from build123d import *

# Parameters (mm, degrees)
FILLET1_R = 0.5


with BuildPart() as part:
    # Sketch1 → Revolve1 (revolve)
    with BuildSketch(Plane.XY):
        with BuildLine():
            Line((10, 0), (10, 26.585564127))
            Line((10, 26.585564127), (1.265397394, 28.234602606))
            Line((1.265397394, 28.234602606), (0, 29.5))
            Line((0, 29.5), (0, 30))
            Line((0, 30), (0.2, 30))
            ThreePointArc((0.2, 30), (0.225652916, 29.998347997), (0.250882045, 29.993419279))
            Line((0.250882045, 29.993419279), (0.8, 29.848964991))
            Line((0.8, 29.848964991), (10.685516518, 27.982641146))
            ThreePointArc((10.685516518, 27.982641146), (11.269907955, 27.638154951), (11.5, 27))
            Line((11.5, 27), (11.5, 0))
            Line((11.5, 0), (10, 0))
        make_face()
    revolve(axis=Axis((0, 9.5, 0), (0, -1, 0)))

    # Fillet1
    fillet1_edges = [part.edges().sort_by_distance(p)[0] for p in [
        (-0.8, 29.848964991, 0),
        (-11.5, 0, 0),
        (-10, 0, 0),
    ]]
    fillet(fillet1_edges, radius=FILLET1_R)


solid = part.part
Geometry: final body of the model. Coordinates: model frame, mm. A direction names the side the tool comes from. Give positions to 0.01 mm unless a question says otherwise; leave off trailing zeros. Write each loop counter-clockwise with the first axis right and the second up, starting at its lowest first coordinate (ties: lowest second). Pieces come first, ordered by that corner, then holes. Notation, with made-up numbers: (10.5, -6) -> (24.5, -6) arc R19 ccw to (24.5, 26) -> close; hole circle Ø3 at (-18.75, 1.25). An arc over 180 degrees is marked (long way). Answer as a JSON object with one key per item and string values.
1. Cut plane A-A on y = 4.5. Output: boundary loops of the cut face in (x, z).
Ans:
{"outline": "circle Ø23 at (0, 0); hole circle Ø20 at (0, 0)"}
2. Contact query for flat-ended pins moving along their axis: pin 1 (4 mm diameter, centred on x = 6.5, z = 6, fed in from +Y); pin 2 (6 mm diameter, centred on x = 4, z = 2.5, fed in from +Y); pin 3 (1.5 mm diameter, centred on x = 3, z = 4, fed in from -Y). Output: stop coordinate, or through.
Ans:
{"pin 1": "stops at y = 28.71", "pin 2": "stops at y = 29.68", "pin 3": "stops at y = 27.39"}
3. Access query for faces 1 (the cylindrical face through (-2.17, 13.73, -9.76)), 2 (the cylindrical face through (-1.5, 13.6, 11.4)). Directions: +Z, -Z, +X, -X, +Y, -Y. A direction counts if a zero-diameter tool reaches every point of the face in a straight line with its end or side. Return the directions, or none.
Ans:
{"face 1": "-Y", "face 2": "+Y, -Y"}
4. Ray query, probe 1 along Z at (x, y) = (0, 9); probe 2 along X at (y, z) = (11.5, -7). Return the intervals inside material, ascending. Write a range as from..to.
Ans:
{"probe 1": "z = -11.5..-10, 10..11.5", "probe 2": "x = -9.12..-7.14, 7.14..9.12"}
5. Mould query, pull axis Z, two halves, no side actions, for faces 3 (the conical face through (0.317, 29.157, -0.131)), 4 (the flat face through (10, 0, -4)), 5 (the conical face through (0.655, 29.732, -1.258)). Classes: pulls with the +Z half, pulls with the -Z half, needs draft (parallel to the pull), parting line crosses it, or undercut.
Ans:
{"face 3": "undercut", "face 4": "needs draft", "face 5": "parting line crosses it"}
